Input: part model. Units: mm. Frame: model coordinates. Face numbers are marked on the shaded views. A direction names the side the tool comes from. Give positions to 0.01 mm unless a question says otherwise; leave off trailing zeros. Write each loop counter-clockwise with the first axis right and the second up, starting at its lowest first coordinate (ties: lowest second). Pieces come first, ordered by that corner, then holes. Notation, with made-up numbers: (-19.75, 12.5) - (22.25, 12.5) arc R21 cw to (22.25, 48.5) - close; hole circle Ø3 at (9, -11). An arc over 180 degrees is marked (long way). Answer as a JSON object with one key per item and string values. Group by question number.
from build123d import *

# Parameters (mm, degrees)
SKETCH2_R          = 5
SKETCH2_R_2        = 3.5
CUT_EXTRUDE1_DEPTH = 0.5


with BuildPart() as part:
    # Sketch1 → Revolve1 (revolve)
    with BuildSketch(Plane.XY):
        Polygon((3, -9.5), (3, 9.5), (5.5, 9.5), (6, 9), (6, 6.75), (5.75, 6.75), (5.75, 5.65), (6, 5.65), (6, -5.65), (5.75, -5.65), (5.75, -6.75), (6, -6.75), (6, -9), (5.5, -9.5), align=None)
    revolve(axis=Axis((0, 9.5, 0), (0, -1, 0)))

    # Sketch2 → Cut-Extrude1 (cut)
    with BuildSketch(Plane(origin=(0, 9.5, 0), x_dir=(1, 0, 0), z_dir=(0, 1, 0))):
        Circle(SKETCH2_R)
        Circle(SKETCH2_R_2, mode=Mode.SUBTRACT)
    cut_extrude1 = extrude(amount=-CUT_EXTRUDE1_DEPTH, mode=Mode.SUBTRACT)

    # Mirror1: Cut-Extrude1 across plane
    add(cut_extrude1.mirror(Plane.ZX), mode=Mode.SUBTRACT)


solid = part.part
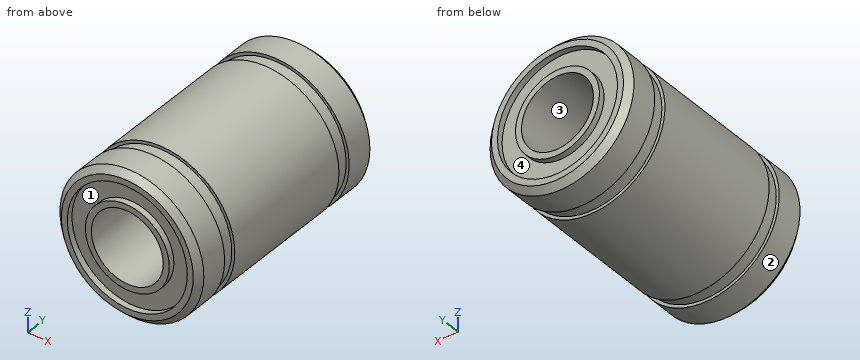
1) Line query: line 1 along Z through (x, y) = (0, 9.35); line 2 along Z through (x, y) = (0, 9.2); line 3 along Y through (x, z) = (4.75, -3.5). Output: solid intervals per line, ascending. Write a range as from..to.
2) Reachability of the marked faces 3 and 4 from +Z, -Z, +X, -X, +Y, -Y: full face, straight path, thin tool, end or side. Return the list, or none.
3) Cut plane A-A on y = 2.5. Return the cut outline in (x, z).
4) Mould query, pull axis Z, two halves, no side actions, for the marked faces 1 and 2. Classes: +Z half, -Z half, draft (parallel to the pull), parting line (faces both ways), or undercut.
5) Cut plane B-B on y = -6. Return the cut outline in (x, z).
6) Pin query (flat end, axial travel): P1, Ø3, axis at y = -4.5, z = 4, coming from the -X side; P2, Ø1.5, axis at y = 7, z = -4, coming from the +X side; P3, Ø5, axis at y = 5.5, z = 4, coming from the -X side. Return the tip coordinate at first contact, or that it passes through.
Filled in:
{
 "1": {"line 1": "z = -5.65..-5, -3.5..-3, 3..3.5, 5..5.65", "line 2": "z = -5.8..-5, -3.5..-3, 3..3.5, 5..5.8", "line 3": "y = -9.1..-6.75, -5.65..5.65, 6.75..9.1"},
 "2": {"face 3": "+Y, -Y", "face 4": "+Y"},
 "3": {"outline": "circle Ø12 at (0, 0); hole circle Ø6 at (0, 0)"},
 "4": {"face 1": "undercut", "face 2": "parting line"},
 "5": {"outline": "circle Ø11.5 at (0, 0); hole circle Ø6 at (0, 0)"},
 "6": {"P1": "stops at x = -5.45", "P2": "stops at x = 5.04", "P3": "stops at x = -5.81"}
}
